Autodesk Inventor part; units mm, degrees
ref_plane "YZ Plane" through (0, 0, 0) normal (1, 0, 0) x (0, 1, 0)
ref_plane "XZ Plane" through (0, 0, 0) normal (0, 1, 0) x (-1, 0, 0)
ref_plane "XY Plane" through (0, 0, 0) normal (0, 0, 1) x (1, 0, 0)
sketch "Sketch1" plane through (0, 0, 0) normal (0, 0, 1) x (1, 0, 0)
  line L0 (-750, 48.3063) -> (750, 48.3063)
  line L1 (750, 48.3063) -> (750, 0)
  line L2 (750, 0) -> (-750, 0)
  line L3 (-750, 0) -> (-750, 48.3063)
  point P0 (0, 0)
  point P1 (0, 0)
  dimension "d0" = 1500
  dimension "d1" = 48.3063
extrude "Plate1" add sketch "Sketch1" along normal blind 3
sketch "Sketch2" plane through (750, 3, 0) normal (0, -1, 0) x (1, 0, 0)
  line L0 (-1500, 0) -> (0, 0)
  line L1 (0, 0) -> (0, 30)
  line L2 (0, 30) -> (-1500, 30)
  line L3 (-1500, 30) -> (-1500, 0)
edge flange "Flange1" height 30 angle 90 thickness 3 bend radius 3 thickness toward (0, -1, 0) relief tear relief width 3 relief depth 1.5 edges at (0, 0, 3) wall of the first edge with corners at (-750, 3, 0) (750, 3, 0) (750, 3, 30) (-750, 3, 30)
bend "Bend1"
corner "Corner1"
sketch "Sketch5" plane through (0, 0, 0) normal (0, 0, -1) x (-1, 0, 0)
  line L0 (750, 48.3063) -> (-750, 48.3063)
  line L1 (500, 48.3063) -> (500, 31)
  line L2 (500, 31) -> (503, 31)
  line L3 (503, 31) -> (503, 48.3063)
  line L4 (750, 0) -> (-750, 0)
  point P0 (0, 0)
  dimension "d18" = 3
  dimension "d19" = 247
  dimension "d20" = 31
extrude "Extrusion1" cut sketch "Sketch5" against normal through all
pattern_linear "Rectangular Pattern1" count 3 spacing 500 along (1, 0, 0) of "Extrusion1"
sketch "Sketch6" plane through (0, 0, 0) normal (0, 0, -1) x (-1, 0, 0)
  line L0 (-750, 48.3063) -> (-750, 6)
  circle A0 centre (-750, 48.3063) radius 15
  line L1 (-750, 48.3063) -> (-500, 48.3063)
  point P0 (0, 0)
  point P1 (-735, 48.3063)
  point P2 (-750, 33.3063)
  dimension "d24" = 30
extrude "Extrusion2" cut sketch "Sketch6" against normal through all contours L1 A0 L0 picked at (-740.1254, 47.1937)
mirror "Mirror1" about plane through (0, 0, 0) normal (1, 0, 0) of "Extrusion2"
equation "\"d1\" = Стрингер_4"
equation "\"d18\" = Thickness"
equation "\"d2\" = Thickness"
equation "\"d3\" = BendReliefWidth"
equation "\"d4\" = BendReliefDepth"
equation "\"d5\" = MinimumRemnant"
equation "\"d6\" = TransitionRadius"
equation "\"d9\" = BendRadius"
equation "\"d10\" = CornerReliefSize"
equation "\"d11\" = GapSize"
equation "\"d12\" = JacobiRadiusSize"
equation "\"BendRadius\" = Thickness"
equation "\"BendReliefWidth\" = Thickness"
equation "\"BendReliefDepth\" = 0.5 * Thickness"
equation "\"CornerReliefSize\" = 4 * Thickness"
equation "\"MinimumRemnant\" = 2 * Thickness"
equation "\"TransitionRadius\" = BendRadius"
equation "\"JacobiRadiusSize\" = BendRadius"
equation "\"GapSize\" = Thickness"
properties part number "МОО 054 стрингер борт 41"
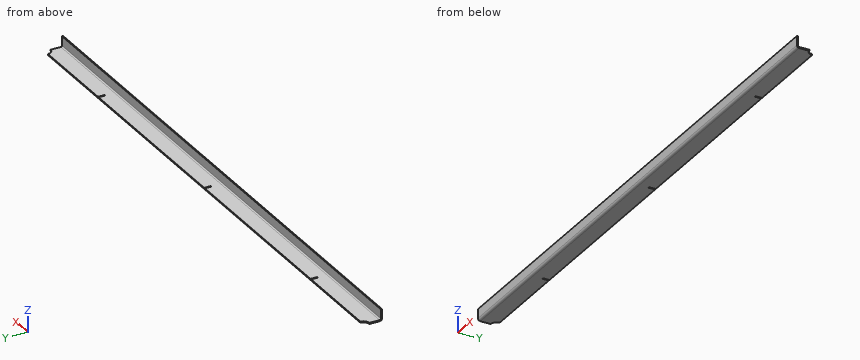
Check sheet for the modelled part. Datum: model origin and axes. Units: mm. Round coordinates to 2 decimals unless told otherwise and drop trailing zeros. Loops run counter-clockwise (first coordinate to the right, second up) from the corner with the lowest first, then second, coordinate; pieces in that order, holes last. Notation, with made-up numbers: (33.5, 11) -> (86.5, 11) arc R25 ccw to (86.5, 24) -> close; hole circle Ø9 at (-30.5, -23). An arc over 180 degrees is marked (long way). Put each result on its own line as item: value. Start each with the question number.
1. Section check A-A (x = 226.5). Enter the section's corners in (y, z).
2. Scan lines: probe 1 along Y at (x, z) = (-525.5, 12.5); probe 2 along Y at (x, z) = (-501, 4). Record each from-to range of solid material in increasing order.
3. Section check B-B (z = 22.75). Enter the section's corners in (x, y), plus the area to 3 significant figures.
4. Gauge pin test, flat ends, axial feed: pin 1 (5 mm diameter, centred on x = -404, y = 10.5, fed in from +Z); pin 2 (0.9 mm diameter, centred on y = 37.5, z = 2, fed in from +X); pin 3 (1.5 mm diameter, centred on y = 35.5, z = 2, fed in from +X). Record the tip position at first contact, or that the pin passes through.
Findings:
1. outline: (0, 6) arc R6 ccw to (6, 0) -> (48.31, 0) -> (48.31, 3) -> (6, 3) arc R3 cw to (3, 6) -> (3, 30) -> (0, 30) -> close
2. probe 1: y = 0 to 3
2. probe 2: y = 0.34 to 3.76
3. outline: (-750, 0) -> (750, 0) -> (750, 3) -> (-750, 3) -> close
3. area: 4,500 mm^2
4. pin 1: stops at z = 3
4. pin 2: stops at x = 740.09
4. pin 3: stops at x = 743.58
